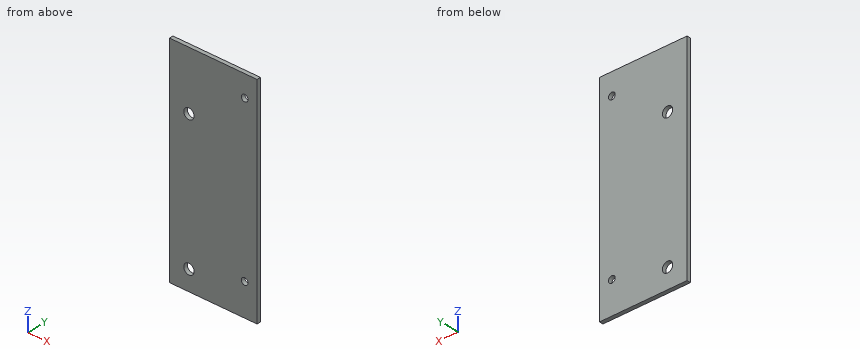
from build123d import *

# Parameters (mm, degrees)
SKETCH1_W               = 57.15
SKETCH1_H               = 140
BOSS_EXTRUDE1_DEPTH     = 2.54
SKETCH2_R               = 2.2
CUT_EXTRUDE1_DEPTH      = 3.54
SKETCH3_R               = 3.3782
CUT_EXTRUDE2_DEPTH      = 1
CUT_EXTRUDE2_DEPTH_BACK = 3.54


with BuildPart() as part:
    # Sketch1 → Boss-Extrude1 (new body)
    with BuildSketch(Plane(origin=(0, 0, 0), x_dir=(1, 0, 0), z_dir=(0, 1, 0))):
        with Locations((28.575, 70)):
            Rectangle(SKETCH1_W, SKETCH1_H)
    extrude(amount=BOSS_EXTRUDE1_DEPTH)

    # Sketch2 → Cut-Extrude1 (cut, through all)
    with BuildSketch(Plane.XZ):
        with Locations((49.1, -119)):
            Circle(SKETCH2_R)
        with Locations((49.1, -14)):
            Circle(SKETCH2_R)
    extrude(amount=-CUT_EXTRUDE1_DEPTH, mode=Mode.SUBTRACT)

    # Sketch3 → Cut-Extrude2 (cut, two sides)
    with BuildSketch(Plane.XZ) as cut_extrude2_sk:
        with Locations((12.7, -127)):
            Circle(SKETCH3_R)
        with Locations((12.7, -38.1)):
            Circle(SKETCH3_R)
    extrude(amount=CUT_EXTRUDE2_DEPTH, mode=Mode.SUBTRACT)
    extrude(cut_extrude2_sk.sketch, amount=-CUT_EXTRUDE2_DEPTH_BACK, mode=Mode.SUBTRACT)


solid = part.part
Check sheet for the modelled part. Datum: model origin and axes. Units: mm. Give positions to 0.01 mm unless a question says otherwise; leave off trailing zeros. Loops run counter-clockwise (first coordinate to the right, second up) from the corner with the lowest first, then second, coordinate; pieces in that order, holes last. Notation, with made-up numbers: M 87,-38 L 123,-38 A28 cw 123,-10 Z; hole C 18,-35 d3. An arc over 180 degrees is marked long. Return JSON: item names as keys, results as strings. Group by question number.
1. Thickness scan on L1, parallel to Z at x = 12.7, y = 2; L2, parallel to Z at x = 49.1, y = 0.65. Record the ranges inside material, lowest first.
2. Cross-section at A-A on x = 12.7. Record the boundary of the cut face in (y, z).
3. Cross-section at B-B on z = -119. Record the boundary of the cut face in (x, y), plus the area to 3 significant figures.
4. Go/stop test with flat-tipped pins: pin 1 (1.5 mm diameter, centred on x = 21.5, z = -93.5, fed in from -Y); pin 2 (6 mm diameter, centred on x = 12.7, z = -127, fed in from +Y). Record where each tip stops, or that it passes through.
Return value:
{
 "1": {"L1": "-140 to -130.38, -123.62 to -41.48, -34.72 to 0", "L2": "-140 to -121.2, -116.8 to -16.2, -11.8 to 0"},
 "2": {"outline": "M 0,-140 L 2.54,-140 L 2.54,-130.38 L 0,-130.38 Z; M 0,-123.62 L 2.54,-123.62 L 2.54,-41.48 L 0,-41.48 Z; M 0,-34.72 L 2.54,-34.72 L 2.54,0 L 0,0 Z"},
 "3": {"outline": "M 0,0 L 46.9,0 L 46.9,2.54 L 0,2.54 Z; M 51.3,0 L 57.15,0 L 57.15,2.54 L 51.3,2.54 Z", "area": "134 mm^2"},
 "4": {"pin 1": "y = 0", "pin 2": "through"}
}
